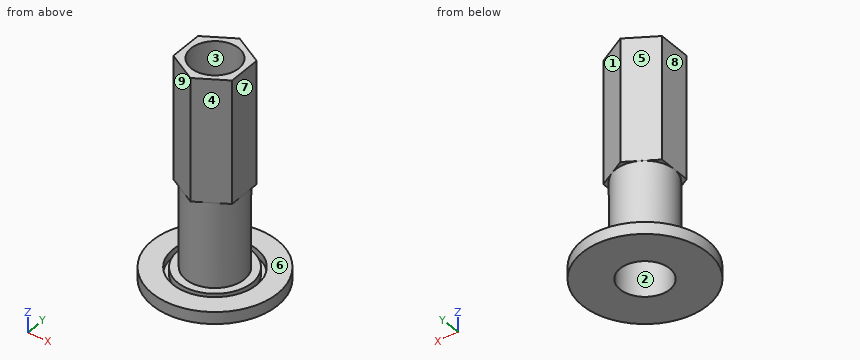
from build123d import *

# Parameters (mm, degrees)
SKETCH2_R           = 16
BOSS_EXTRUDE1_DEPTH = 82.25


with BuildPart() as part:
    # Sketch1 → Revolve1 (revolve)
    with BuildSketch(Plane(origin=(0, 0, 0), x_dir=(1, 0, 0), z_dir=(0, 1, 0))):
        Polygon((0, 0), (16, 0), (16, -71), (19.65, -71), (19.65, 68), (24.95, 68), (24.95, 73), (28.1, 73), (28.1, 68), (42, 68), (42, 76), (16.65, 76), (16.65, 18.004366875), (12, 18.004366875), (12, 24.882682167), (0, 24.882682167), align=None)
    revolve(axis=Axis((0, 0, 39.840023079), (0, 0, -1)))

    # Sketch2 → Boss-Extrude1 (add)
    with BuildSketch(Plane.XY.offset(71)):
        Polygon((0, 22.689865579), (-19.65, 11.34493279), (-19.65, -11.34493279), (0, -22.689865579), (19.65, -11.34493279), (19.65, 11.34493279), align=None)
        Circle(SKETCH2_R, mode=Mode.SUBTRACT)
    extrude(amount=-BOSS_EXTRUDE1_DEPTH)


solid = part.part
CAD build for the part. Positions are in the model's coordinates, mm. Face numbers are marked on the shaded views. A direction names the side the tool comes from. Round coordinates to 2 decimals unless told otherwise and drop trailing zeros. Loops run counter-clockwise (first coordinate to the right, second up) from the corner with the lowest first, then second, coordinate; pieces in that order, holes last.
(1) Which spindle directions (+Z, -Z, +X, -X, +Y, -Y) get a long thin tool onto all of the face, cutting with end or side? Do the marked faces 5, 6, 7, 8 and 9. Say none if no direction does.
(2) Cut at A-A (z = 40). Give the cut face in (x, y).
(3) Two-plate mould, pull along Y, no slides. Class the marked faces 1, 2, 3 and 4: +Y half, -Y half, draft (parallel to the pull), parting line (faces both ways), or undercut.
(4) Cut at B-B (x = -14). Give the cut face in (y, z).
(5) Wall check: line 1 along Y through (x, z) = (0, 38); line 2 along Y through (x, z) = (0, -59); line 3 along X through (y, z) = (0, 46). Give the ranges that are in metal, low to high.
(6) Cut at C-C (y = -35.5). Give the cut face in (x, z), plus the area to 3 significant figures.
(7) Drop flat-ended pins along their axis: pin 1 (3 mm diameter, centred on x = 12.5, y = 8, fed in from -Z); pin 2 (1 mm diameter, centred on y = -16.5, z = 36.5, fed in from +X); pin 3 (11.5 mm diameter, centred on y = 3, z = 12.5, fed in from +X). Give the stop position or say it passes through.
Findings below:
1. face 5: +Z, -X, +Y
1. face 6: +Z
1. face 7: +Z, +X, +Y, -Y
1. face 8: +Z, -X, +Y, -Y
1. face 9: +Z, -X, -Y
2. outline: (-19.65, -11.34) - (0, -22.69) - (19.65, -11.34) - (19.65, 11.34) - (0, 22.69) - (-19.65, 11.34) - close; hole circle Ø32 at (0, 0)
3. face 1: +Y half
3. face 2: undercut
3. face 3: undercut
3. face 4: -Y half
4. outline: (-39.6, -76) - (-9.01, -76) - (-9.01, -18) - (9.01, -18) - (9.01, -76) - (39.6, -76) - (39.6, -68) - (24.36, -68) - (24.36, -73) - (20.65, -73) - (20.65, -68) - (13.79, -68) - (13.79, -11.25) - (14.61, -11.25) - (14.61, 71) - (7.75, 71) - (7.75, 0) - (-7.75, 0) - (-7.75, 71) - (-14.61, 71) - (-14.61, -11.25) - (-13.79, -11.25) - (-13.79, -68) - (-20.65, -68) - (-20.65, -73) - (-24.36, -73) - (-24.36, -68) - (-39.6, -68) - close
5. line 1: y = -22.69 to -16, 16 to 22.69
5. line 2: y = -19.65 to -16.65, 16.65 to 19.65
5. line 3: x = -19.65 to -16, 16 to 19.65
6. outline: (-22.44, -76) - (22.44, -76) - (22.44, -68) - (-22.44, -68) - close
6. area: 359 mm2
7. pin 1: stops at z = -18
7. pin 2: stops at x = 11.59
7. pin 3: stops at x = 19.65
